Here's the drawing with two shaded views (mm, measured from the low corner). I have some questions. Coordinates: 2 decimals unless noted, no trailing zeros. Loops run counter-clockwise (first coordinate to the right, second up) from the corner with the lowest first, then second, coordinate; pieces in that order, holes last. Notation, with made-up numbers: M -39.5,40 L -4.5,40 A19 cw -4.5,56 Z; hole C -39.75,62 d10. An arc over 180 degrees is marked long. Return JSON: item names as keys, results as strings. Group by question number.
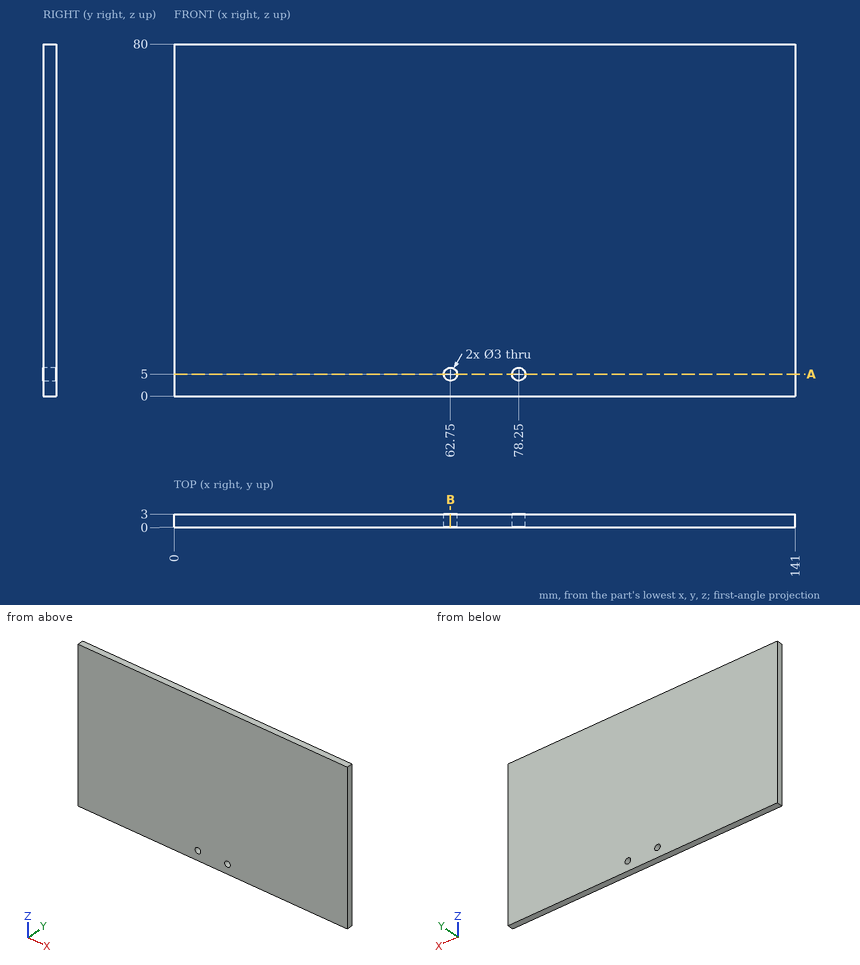
(1) Imagine slicing it at A-A, the plane z = 5. Write out the boundary of the cut face in (x, y), then the cut area to 3 significant figures.
(2) Imagine slicing it at B-B, the plane x = 62.75. Write out the boundary of the cut face in (y, z), then the cut area to 3 significant figures.
(3) If I drill on L1, parallel to X at y = 0.75, z = 5; L2, parallel to Z at x = 78.25, y = 1.4; L3, parallel to Z at x = 77.5, y = 0.95, over which ranges is the centre line in solid material (lowest first)? Write a range as [from, to].
(4) Will this pin go through, and if not, where does the flat tip stop? P1, Ø2.5, axis at x = 62.75, z = 5, coming from the -Y side.
Checks:
{
 "1": {"outline": "M 0,0 L 61.25,0 L 61.25,3 L 0,3 Z; M 64.25,0 L 76.75,0 L 76.75,3 L 64.25,3 Z; M 79.75,0 L 141,0 L 141,3 L 79.75,3 Z", "area": "405 mm²"},
 "2": {"outline": "M 0,0 L 3,0 L 3,3.5 L 0,3.5 Z; M 0,6.5 L 3,6.5 L 3,80 L 0,80 Z", "area": "231 mm²"},
 "3": {"L1": "[0, 61.25], [64.25, 76.75], [79.75, 141]", "L2": "[0, 3.5], [6.5, 80]", "L3": "[0, 3.7], [6.3, 80]"},
 "4": {"P1": "through"}
}
